Could you check a few things on this model? Use its own coordinates, in mm. A direction names the side the tool comes from. Coordinates: 2 decimals unless noted, no trailing zeros. Write each loop counter-clockwise with the first axis right and the second up, starting at its lowest first coordinate (ties: lowest second). Pieces come first, ordered by that corner, then holes. Notation, with made-up numbers: M -32.75,-0.75 L 15.25,-0.75 A17 cw 15.25,13.25 Z; hole C 32.25,27.5 d4. An arc over 180 degrees is marked long. Write item = value, one per line.
```python
from build123d import *


with BuildPart() as part:
    # Эскиз1 → Повернуть1 (revolve)
    with BuildSketch(Plane.XY, mode=Mode.PRIVATE) as revolve_1_sk:
        with BuildLine():
            Line((6, 20), (-6, 20))
            ThreePointArc((-6, 20), (-7.060660172, 20.439339828), (-7.5, 21.5))
            Line((-7.5, 21.5), (-7.5, 25.166666667))
            Line((-7.5, 25.166666667), (-5, 25.166666667))
            Line((-5, 25.166666667), (-5, 28.833333333))
            Line((-5, 28.833333333), (-7.5, 28.833333333))
            Line((-7.5, 28.833333333), (-7.5, 32.5))
            ThreePointArc((-7.5, 32.5), (-7.060660172, 33.560660172), (-6, 34))
            Line((-6, 34), (6, 34))
            ThreePointArc((6, 34), (7.060660172, 33.560660172), (7.5, 32.5))
            Line((7.5, 32.5), (7.5, 28.833333333))
            Line((7.5, 28.833333333), (5, 28.833333333))
            Line((5, 28.833333333), (5, 25.166666667))
            Line((5, 25.166666667), (7.5, 25.166666667))
            Line((7.5, 25.166666667), (7.5, 21.5))
            ThreePointArc((7.5, 21.5), (7.060660172, 20.439339828), (6, 20))
        make_face()
    revolve(revolve_1_sk.sketch.rotate(Axis((-1000, 0, 0), (1, 0, 0)), 90), axis=Axis((-1000, 0, 0), (1, 0, 0)))


solid = part.part
```
Item 1: I'm going to push flat-ended pins straight in: P1, Ø1, axis at x = 5.5, y = 17, coming from the +Z side; P2, Ø17.5, axis at y = 2, z = -3.5, coming from the -X side; P3, Ø2, axis at x = 5.5, z = 2, coming from the +Y side; P4, Ø3, axis at y = -0.5, z = 19, coming from the -X side. Where does each tip first touch, or does it pass through?
Numbers:
P1 = 29.73
P2 = through
P3 = 33.99
P4 = -7.12
Item 2: Imagine slicing it at C-C (x = -2.5). Write out the boundary of the cut face in (y, z), and give its area (3 significant figures).
Numbers:
outline = C 0,0 d68; hole C 0,0 d40
area = 2,380 mm²
Item 3: For faces 4 (the face through (-0.08, -0.88, -19.98)), 5 (the face through (5, -24, -9)), 6 (the face through (-6.232, 15.314, -19.971)), which set-ups out of +Z, -Z, +X, -X, +Y, -Y let a thin tool reach every point of the face, with its end or its side?
Numbers:
face_4 = +X, -X
face_5 = +X
face_6 = -X
Item 4: If I drill on line 1 along Y through (x, z) = (5.75, 0); line 2 along Y through (x, z) = (-6.65, 0); line 3 along Y through (x, z) = (-1.5, 0), over which ranges is the centre line in solid material (lowest first)?
Numbers:
line_1 = -34 to -28.83, -25.17 to -20, 20 to 25.17, 28.83 to 34
line_2 = -33.85 to -28.83, -25.17 to -20.15, 20.15 to 25.17, 28.83 to 33.85
line_3 = -34 to -20, 20 to 34
Item 5: If we mould it in two halves opening along Z, with no side actions, what happens to faces 1 (the face through (0.08, -33.71, -4.43)), 2 (the face through (6.23, -19.49, -21.25)), 3 (the face through (7.5, 26.3, -12.2))? For each: pulls with the +Z half, pulls with the -Z half, needs draft (parallel to the pull), parting line crosses it, or undercut.
Numbers:
face_1 = parting line crosses it
face_2 = undercut
face_3 = needs draft
